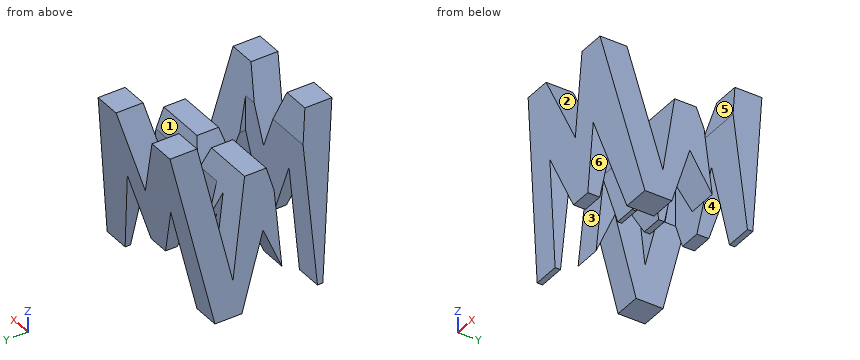
from build123d import *

# Parameters (mm, degrees)
F0_W      = 38.1
F0_H      = 38.1
F1_DEPTH  = 38.1
F6_DEPTH  = 38.1
F8_DEPTH  = 38.1
F9_W      = 25.4
F9_H      = 7.62
F10_DEPTH = 38.1


with BuildPart() as f1:
    # F0 (on Front) → F1 (new body)
    with BuildSketch(Plane.XZ):
        with Locations((19.05, 19.05)):
            Rectangle(F0_W, F0_H)
    extrude(amount=F1_DEPTH)

    # F5 (on offset) → F6 (cut)
    with BuildSketch(Plane.YZ.offset(38.1)):
        Polygon((-11.43, 7.62), (-6.35, 38.1), (-31.75, 38.1), (-26.67, 7.62), (-21.59, 28.575), (-16.51, 28.575), align=None)
        Polygon((-31.75, 0), (-38.1, 38.1), (-38.1, 0), align=None)
        Polygon((-25.4, 0), (-12.7, 0), (-19.427248, 15.875), align=None)
        Polygon((-6.35, 0), (0, 0), (0, 38.1), align=None)
    extrude(amount=-F6_DEPTH, mode=Mode.SUBTRACT)

    # F7 (on offset) → F8 (cut)
    with BuildSketch(Plane.XZ.offset(38.1)):
        Polygon((10.054167, 22.225), (6.35, 0), (31.75, 0), (25.4, 22.225), (20.214167, 9.260417), (15.134167, 9.260417), align=None)
        Polygon((0, 38.1), (0, 0), (6.35, 38.1), align=None)
        Polygon((25.4, 38.1), (12.7, 38.1), (19.05, 22.225), align=None)
        Polygon((31.75, 38.1), (38.1, 0), (38.1, 38.1), align=None)
    extrude(amount=-F8_DEPTH, mode=Mode.SUBTRACT)

    # F9 (on offset) → F10 (cut)
    with BuildSketch(Plane.XY.offset(38.1)):
        with Locations((25.4, -11.43)):
            Rectangle(F9_W, F9_H)
        with Locations((12.7, -26.67)):
            Rectangle(F9_W, F9_H)
    extrude(amount=-F10_DEPTH, mode=Mode.SUBTRACT)


solid = f1.part
Can you work these out from the model? Positions are in its coordinate system, mm. Face numbers are marked on the shaded views. A direction names the side the tool comes from. Give positions to 0.01 mm unless a question says otherwise; leave off trailing zeros. Order: outer loops, then holes, each group sorted by start corner. A loop starts at its lowest first (then second) coordinate and runs counter-clockwise, first axis right, second up. Notation, with made-up numbers: M 78.5,55 L 87.5,55 A14 cw 87.5,76 Z; hole C -12.5,-22.5 d7. An arc over 180 degrees is marked long. Use a Markdown table: item, result. Add a question column.
Item 1: Suppose I cut it at B-B (x = 26). List the corners of the cut face in (y, z) for me (3 decimals).
Item 2: For the marked faces 1, 2, 3 and 4, which set-ups out of +Z, -Z, +X, -X, +Y, -Y let a thin tool reach every point of the face, with its end or its side?
Item 3: If I drill on L1, parallel to Y at x = 4.5, z = 9; L2, parallel to Y at x = 29, z = 20; L3, parallel to X at y = -18, z = 15.5, over which ranges is the centre line in solid material (lowest first)? Write a range as [from, to].
Item 4: Suppose I cut it at A-A (z = 31.5). List the corners of the cut face in (x, y) for me, then the cut area to 3 significant figures.
Item 5: Will these pins go through, and if not, where does the flat tip stop? pin 1 (1.4 mm diameter, centred on x = 19, y = -6, fed in from -Z); pin 2 (0.8 mm diameter, centred on y = -8.5, z = 26, fed in from +X); pin 3 (8 mm diameter, centred on y = -9.5, z = 20, fed in from +X); pin 4 (4 mm diameter, centred on y = -25.5, z = 23.5, fed in from -X).
Item 6: Suppose I cut it at C-C (y = -32.5). List the corners of the cut face in (x, z) for me (3 decimals), then the cut area to 3 significant figures.
Item 7: We'd pull the mould along Y, two halves only. Please class the marked faces 5 and 6: +Y half, -Y half, draft (parallel to the pull), parting line (faces both ways), or undercut.
Answer sheet:
| question | item | result |
|---|---|---|
| 1 | outline | M -38.1,38.1 L -35.104,20.125 L -28.754,20.125 L -31.75,38.1 Z; M -23.638,20.125 L -15.24,20.125 L -15.24,23.336 L -16.51,28.575 L -21.59,28.575 Z; M -7.62,20.125 L -2.996,20.125 L 0,38.1 L -6.35,38.1 L -7.62,30.48 Z |
| 2 | face 1 | +Z, +X, -X |
| 2 | face 2 | +Z, +Y, -Y |
| 2 | face 3 | +Z, -Z, -X |
| 2 | face 4 | -Z, +Y, -Y |
| 3 | L1 | y = [-33.25, -30.48], [-22.86, -22.01], [-16.51, -11.76], [-11.2, -4.85] |
| 3 | L2 | y = [-35.08, -28.73], [-23.67, -15.24], [-7.62, -3.02] |
| 3 | L3 | x = [2.58, 8.93], [12.69, 22.71], [27.32, 35.52] |
| 4 | outline | M 5.25,-37 L 15.34,-37 L 15.34,-30.65 L 5.25,-30.65 Z; M 5.25,-7.45 L 15.34,-7.45 L 15.34,-1.1 L 5.25,-1.1 Z; M 22.76,-37 L 32.85,-37 L 32.85,-30.65 L 22.76,-30.65 Z; M 22.76,-7.45 L 32.85,-7.45 L 32.85,-1.1 L 22.76,-1.1 Z |
| 4 | area | 256 mm² |
| 5 | pin 1 | stops at z = 9.26 |
| 5 | pin 2 | stops at x = 12.7 |
| 5 | pin 3 | stops at x = 35.36 |
| 5 | pin 4 | passes through |
| 6 | outline | M 0.75,4.5 L 7.1,4.5 L 10.054,22.225 L 15.134,9.26 L 20.214,9.26 L 25.4,22.225 L 30.464,4.5 L 37.35,4.5 L 31.75,38.1 L 25.4,38.1 L 19.05,22.225 L 12.7,38.1 L 6.35,38.1 Z |
| 6 | area | 730 mm² |
| 7 | face 5 | undercut |
| 7 | face 6 | draft |
